Could you check a few things on this model? Use its own coordinates, in mm. A direction names the side the tool comes from. Coordinates: 2 decimals unless noted, no trailing zeros. Order: outer loops, then holes, each group sorted by start corner. A loop starts at its lowest first (then second) coordinate and runs counter-clockwise, first axis right, second up. Notation, with made-up numbers: (-9.75, 88.5) -> (46.25, 88.5) arc R28 cw to (46.25, 109.5) -> close; hole circle Ø3 at (20, 52.5). An arc over 180 degrees is marked (long way). Use a Markdown table: item, result. Add a question column.
1) Will these pins go through, and if not, where does the flat tip stop? pin 1 Ø1 at (x, y) = (-1.5, 4) entering from +Z; pin 2 Ø3.5 at (y, z) = (-2, 10) entering from +X (3 decimals); pin 3 Ø3 at (x, y) = (0, 0) entering from -Z; pin 4 Ø5 at (x, z) = (-3.5, 16.5) entering from -Y (3 decimals).
2) If I drill on L1, parallel to X at y = 0, z = -1.05 (1 decimal); L2, parallel to X at y = 0, z = 12.25 (3 decimals); L3, parallel to Y at x = 0, z = 24.6 (3 decimals), over which ranges is the centre line in solid material (lowest first)? Write a range as [from, to].
3) Which directions (+Z, -Z, +X, -X, +Y, -Y) give clear straight access to the entire face, cutting with the end or side of a thin tool? Please do faces 4 (the cylindrical face through (-6.623, 6.603, 12.878)), 5 (the flat face through (0, -6.985, 13)), 6 (the flat face through (0, 6.985, 13)).
4) If we section it at A-A (y = 0): Write out the boundary of the cut face in (x, z) (1 decimal), plus the area to 3 significant figures.
5) If we section it at C-C (z = 10.25): Write out the boundary of the cut face in (x, y) (3 decimals), plus the area to 3 significant figures.
6) If we section it at D-D (x = -5): Write out the boundary of the cut face in (y, z) (1 decimal), plus the area to 3 significant figures.
7) Thinking about a two-plate mould opening in X: for faces 1 (the cylindrical face through (5.45, 1.72, 24.15)), 2 (the flat face through (-6, 0, 25.4)), 3 (the flat face through (7.938, 0, -1)), which applies, +X half, -X half, draft (parallel to the pull), parting line (faces both ways), or undercut?
```python
from build123d import *

# Parameters (mm, degrees)
F0_W           = 13.97
F0_H           = 13.97
F1_DEPTH       = 25.4
F2_R           = 5.715
F3_DEPTH       = 2.54
F5_R           = 1.27
F6_W           = 15.875
F6_H           = 15.875
F7_DEPTH       = 2.54
F8_R           = 1.27
F9_R           = 0.762
F4_R           = 1.905
F10_DEPTH      = 25.401
F10_DEPTH_BACK = 2.541


with BuildPart() as f1:
    # F0 (on Top) → F1 (new body)
    with BuildSketch(Plane.XY):
        Rectangle(F0_W, F0_H)
    extrude(amount=F1_DEPTH)

    # F2 (on face) → F3 (cut)
    with BuildSketch(Plane.XY.offset(25.4)):
        Circle(F2_R)
    extrude(amount=-F3_DEPTH, mode=Mode.SUBTRACT)

    # F5
    f5_edges = [f1.edges().sort_by_distance(p)[0] for p in [
        (-6.985, 6.985, 12.7),
        (-6.985, -6.985, 12.7),
        (6.985, 6.985, 12.7),
        (6.985, -6.985, 12.7),
    ]]
    fillet(f5_edges, radius=F5_R)

    # F6 (on face) → F7 (join)
    with BuildSketch(Plane(origin=(0, 0, 0), x_dir=(1, 0, 0), z_dir=(0, 0, -1))):
        Rectangle(F6_W, F6_H)
    extrude(amount=F7_DEPTH)

    # F8
    f8_edges = [f1.edges().sort_by_distance(p)[0] for p in [
        (7.9375, -7.9375, -1.27),
        (-7.9375, -7.9375, -1.27),
        (-7.9375, 7.9375, -1.27),
        (7.9375, 7.9375, -1.27),
    ]]
    fillet(f8_edges, radius=F8_R)

    # F9
    f9_edges = [f1.edges().sort_by_distance(p)[0] for p in [
        (0, -7.9375, -2.54),
    ]]
    fillet(f9_edges, radius=F9_R)

    # F4 (on face) → F10 (cut, two sides)
    with BuildSketch(Plane(origin=(0, 0, 0), x_dir=(1, 0, 0), z_dir=(0, 0, -1))) as f10_sk:
        Circle(F4_R)
    extrude(amount=-F10_DEPTH, mode=Mode.SUBTRACT)
    extrude(f10_sk.sketch, amount=F10_DEPTH_BACK, mode=Mode.SUBTRACT)


solid = f1.part
```
Answer sheet:
| question | item | result |
|---|---|---|
| 1 | pin 1 | z = 22.86 |
| 1 | pin 2 | x = 6.985 |
| 1 | pin 3 | through |
| 1 | pin 4 | y = -6.985 |
| 2 | L1 | [-7.9, -1.9], [1.9, 7.9] |
| 2 | L2 | [-6.985, -1.905], [1.905, 6.985] |
| 2 | L3 | [-6.985, -5.715], [5.715, 6.985] |
| 3 | face 4 | +Z, -X, +Y |
| 3 | face 5 | +Z, +X, -X, -Y |
| 3 | face 6 | +Z, +X, -X, +Y |
| 4 | outline | (-7.9, -1.8) arc R0.8 ccw to (-7.2, -2.5) -> (-1.9, -2.5) -> (-1.9, 22.9) -> (-5.7, 22.9) -> (-5.7, 25.4) -> (-7, 25.4) -> (-7, 0) -> (-7.9, 0) -> close; (1.9, -2.5) -> (7.2, -2.5) arc R0.8 ccw to (7.9, -1.8) -> (7.9, 0) -> (7, 0) -> (7, 25.4) -> (5.7, 25.4) -> (5.7, 22.9) -> (1.9, 22.9) -> close |
| 4 | area | 269 mm2 |
| 5 | outline | (-6.985, -5.715) arc R1.27 ccw to (-5.715, -6.985) -> (5.715, -6.985) arc R1.27 ccw to (6.985, -5.715) -> (6.985, 5.715) arc R1.27 ccw to (5.715, 6.985) -> (-5.715, 6.985) arc R1.27 ccw to (-6.985, 5.715) -> close; hole circle Ø3.81 at (0, 0) |
| 5 | area | 182 mm2 |
| 6 | outline | (-7.9, -1.8) arc R0.8 ccw to (-7.2, -2.5) -> (7.2, -2.5) arc R0.8 ccw to (7.9, -1.8) -> (7.9, 0) -> (7, 0) -> (7, 25.4) -> (2.8, 25.4) -> (2.8, 22.9) -> (-2.8, 22.9) -> (-2.8, 25.4) -> (-7, 25.4) -> (-7, 0) -> (-7.9, 0) -> close |
| 6 | area | 381 mm2 |
| 7 | face 1 | undercut |
| 7 | face 2 | draft |
| 7 | face 3 | +X half |
